Autodesk Inventor part; units mm, degrees
ref_plane "YZ Plane" through (0, 0, 0) normal (1, 0, 0) x (0, 1, 0)
ref_plane "XZ Plane" through (0, 0, 0) normal (0, 1, 0) x (-1, 0, 0)
ref_plane "XY Plane" through (0, 0, 0) normal (0, 0, 1) x (1, 0, 0)
sketch "スケッチ1" plane through (0, 0, 0) normal (0, 0, 1) x (1, 0, 0)
  line L0 (0, 10) -> (11.5, 10)
  line L1 (7.1451, -0.8872) -> (11.5, 10)
  line L2 (0, 10) -> (0, 0) construction
  line L3 (0, 10) -> (-11.5, 10)
  line L4 (-7.1451, -0.8872) -> (-11.5, 10)
  line L5 (7.1451, -0.8872) -> (7.1451, -45.8872)
  line L6 (-7.1451, -45.8872) -> (-7.1451, -0.8872)
  line L7 (-7.1451, -23.3872) -> (7.1451, -23.3872) construction
  line L8 (0, -56.7743) -> (11.5, -56.7743)
  line L9 (7.1451, -45.8872) -> (11.5, -56.7743)
  line L10 (0, -56.7743) -> (-11.5, -56.7743)
  line L11 (-7.1451, -45.8872) -> (-11.5, -56.7743)
  line L12 (7.1451, -0.8872) -> (7.1451, -45.8872)
  line L13 (7.1451, -45.8872) -> (11.5, -56.7743)
  line L14 (11.5, -56.7743) -> (-11.5, -56.7743)
  line L15 (-11.5, -56.7743) -> (-7.1451, -45.8872)
  line L16 (-7.1451, -45.8872) -> (-7.1451, -0.8872)
  line L17 (-7.1451, -0.8872) -> (-11.5, 10)
  line L18 (-11.5, 10) -> (11.5, 10)
  line L19 (11.5, 10) -> (7.1451, -0.8872)
  dimension "d0" = 7.2
  dimension "d1" = 11.5
  dimension "d3" = 45
extrude "押し出し1" add sketch "スケッチ1" along normal blind 3.8
sketch "スケッチ2" plane through (0, 0, 3.8) normal (0, 0, 1) x (1, 0, 0)
  line L0 (-11.5, 10) -> (-7.1451, -0.8872)
  line L1 (-7.1451, -0.8872) -> (-14.6451, -0.8872)
  line L2 (-14.6451, -0.8872) -> (-14.6451, -45.8872)
  line L3 (-14.6451, -45.8872) -> (-7.1451, -45.8872)
  line L4 (-7.1451, -45.8872) -> (-7.1451, -0.8872)
  line L5 (7.1451, -45.8872) -> (7.1451, -0.8872)
  line L6 (7.1451, -0.8872) -> (14.6451, -0.8872)
  line L7 (14.6451, -0.8872) -> (14.6451, -45.8872)
  line L8 (14.6451, -45.8872) -> (7.1451, -45.8872)
  line L9 (7.1451, -45.8872) -> (7.1451, -0.8872)
  point P0 (0, 0)
  dimension "d6" = 7.5
  dimension "d7" = 45
  dimension "d8" = 7.5
extrude "押し出し2" add sketch "スケッチ2" against normal blind 3.8
sketch "スケッチ3" plane through (0, 0, 3.8) normal (0, 0, 1) x (1, 0, 0)
  line L0 (14.6451, -0.8872) -> (14.6451, -45.8872)
  line L1 (-7.1451, -45.8872) -> (-14.6451, -45.8872)
  line L2 (14.6451, -0.8872) -> (-14.6451, -0.8872)
  line L3 (-14.6451, -0.8872) -> (-14.6451, -45.8872)
  line L4 (-14.6451, -45.8872) -> (14.6451, -45.8872)
  line L5 (14.6451, -45.8872) -> (14.6451, -0.8872)
  point P0 (0, 0)
extrude "押し出し3" add sketch "スケッチ3" along normal blind 3
properties part number "iPad_mount_center"
Design review of the part built by this model. Coordinates are the model's own, in mm. A direction names the side the tool comes from. Round coordinates to 2 decimals unless told otherwise and drop trailing zeros. Write each loop counter-clockwise with the first axis right and the second up, starting at its lowest first coordinate (ties: lowest second). Pieces come first, ordered by that corner, then holes.
Item 1: The part is to be moulded in two halves that separate along Y. For faces 4 (the flat face through (-14.645, -23, 3)), 5 (the flat face through (9.29, -51.25, 1.87)), 6 (the flat face through (0, 10, 2)), 7 (the flat face through (0, -56.774, 2)), say which applies: +Y half, -Y half, draft (parallel to the pull), parting line (faces both ways), or undercut.
Item 2: We need section C-C on x = -5.5. Write out the cut boundary in (y, z).
Item 3: We need section A-A on z = 2. Write out the cut boundary in (x, y), and give its area (3 significant figures).
Item 4: We need section D-D on x = -9.25. Write out the cut boundary in (y, z).
Item 5: For probe 1 along Y at (x, z) = (9.75, 3.5); probe 2 along Y at (x, z) = (-2.25, 5.75); probe 3 along Z at (x, y) = (-6.75, -48.5), list the stretches that pass through material, from the lowest coordinate up.
Item 6: We need section B-B on x = 8.75. Write out the cut boundary in (y, z), and give its area (3 significant figures).
Item 7: Clearance check with flat-ended pins moving along their axes: pin 1 Ø4 at (y, z) = (1.5, 3) entering from +X; pin 2 Ø2 at (x, z) = (7, 5) entering from +Y. State where each tip first meets the part, or that it passes through.
Item 8: For faces 1 (the flat face through (9.3, 4.5, 1.9)), 2 (the flat face through (0, -51, 3.8)), 3 (the flat face through (-9.29, -51.25, 1.87)), list the 3-axis set-ups (+Z, -Z, +X, -X, +Y, -Y) from which the entire face can be reached by the end or side of a thin tool; tool diameter is ignored.
Returned:
1. face 4: draft
1. face 5: undercut
1. face 6: +Y half
1. face 7: -Y half
2. outline: (-56.77, 0) - (10, 0) - (10, 3.8) - (-0.89, 3.8) - (-0.89, 6.8) - (-45.89, 6.8) - (-45.89, 3.8) - (-56.77, 3.8) - close
3. outline: (-14.65, -45.89) - (-7.15, -45.89) - (-11.5, -56.77) - (11.5, -56.77) - (7.15, -45.89) - (14.65, -45.89) - (14.65, -0.89) - (7.15, -0.89) - (11.5, 10) - (-11.5, 10) - (-7.15, -0.89) - (-14.65, -0.89) - close
3. area: 1,720 mm2
4. outline: (-56.77, 0) - (-51.15, 0) - (-51.15, 3.8) - (-56.77, 3.8) - close; (-45.89, 0) - (-0.89, 0) - (-0.89, 6.8) - (-45.89, 6.8) - close; (4.38, 0) - (10, 0) - (10, 3.8) - (4.38, 3.8) - close
5. probe 1: y = -56.77 to -52.4, -45.89 to -0.89, 5.63 to 10
5. probe 2: y = -45.89 to -0.89
5. probe 3: z = 0 to 3.8
6. outline: (-56.77, 0) - (-49.9, 0) - (-49.9, 3.8) - (-56.77, 3.8) - close; (-45.89, 0) - (-0.89, 0) - (-0.89, 6.8) - (-45.89, 6.8) - close; (3.13, 0) - (10, 0) - (10, 3.8) - (3.13, 3.8) - close
6. area: 358 mm2
7. pin 1: stops at x = 8.9
7. pin 2: stops at y = -0.89
8. face 1: +Z, -Z, +X
8. face 2: +Z, +X, -X, -Y
8. face 3: +Z, -Z, -X
